from build123d import *

# Parameters (mm, degrees)
SKETCH1_W              = 55
SKETCH1_H              = 20
BOSS_EXTRUDE2_DEPTH    = 40
FILLET3_R              = 27.5
SKETCH3_R              = 10.2
CUT_EXTRUDE1_DEPTH     = 40
SKETCH4_R              = 1.5
CUT_EXTRUDE2_DEPTH     = 40
CUT_EXTRUDE3_OUTLINE_W = 1.013964341
CUT_EXTRUDE3_OUTLINE_H = 3.461369181
CUT_EXTRUDE4_OUTLINE_W = 1.011767624
CUT_EXTRUDE4_OUTLINE_H = 3.485879142


# Read off the part's stored shape, not the designer's step: Cut-Extrude3, Cut-Extrude4
with BuildPart() as part:
    # Sketch1 → Boss-Extrude2 (new body)
    with BuildSketch(Plane(origin=(0, 0, 0), x_dir=(1, 0, 0), z_dir=(0, 1, 0))):
        Rectangle(SKETCH1_W, SKETCH1_H)
    extrude(amount=BOSS_EXTRUDE2_DEPTH)

    # Fillet3
    fillet3_edges = [part.edges().sort_by_distance(p)[0] for p in [
        (27.5, 40, 0),
        (-27.5, 40, 0),
    ]]
    fillet(fillet3_edges, radius=FILLET3_R - 0.0001)  # a hair under: the kernel refuses the full size

    # Sketch3 → Cut-Extrude1 (cut)
    with BuildSketch(Plane(origin=(0, 0, -10), x_dir=(-1, 0, 0), z_dir=(0, 0, -1))):
        with Locations((0, 20)):
            Circle(SKETCH3_R)
    extrude(amount=-CUT_EXTRUDE1_DEPTH, mode=Mode.SUBTRACT)

    # Sketch4 → Cut-Extrude2 (cut)
    with BuildSketch(Plane.XZ):
        with Locations(Location((-11.5, 0, 0), (0, 0, 270))):
            Circle(SKETCH4_R)
        with Locations(Location((11.5, 0, 0), (0, 0, 270))):
            Circle(SKETCH4_R)
    extrude(amount=-CUT_EXTRUDE2_DEPTH, mode=Mode.SUBTRACT)

    # Cut-Extrude3 outline → Cut-Extrude3 (revolve, cut)
    with BuildSketch(Plane(origin=(11.536337156, 0, 0.030463059), x_dir=(1, 0, 0), z_dir=(0, 0, 1))):
        with Locations((1.959565013, 36.730684591)):
            Rectangle(CUT_EXTRUDE3_OUTLINE_W, CUT_EXTRUDE3_OUTLINE_H)
    revolve(axis=Axis((11.536337156, 0, 0.030463059), (0, 1, 0)), mode=Mode.SUBTRACT)

    # Cut-Extrude4 outline → Cut-Extrude4 (revolve, cut)
    with BuildSketch(Plane(origin=(-11.463662844, 0, 0.030463059), x_dir=(1, 0, 0), z_dir=(0, 0, 1))):
        with Locations((1.958466654, 36.742939571)):
            Rectangle(CUT_EXTRUDE4_OUTLINE_W, CUT_EXTRUDE4_OUTLINE_H)
    revolve(axis=Axis((-11.463662844, 0, 0.030463059), (0, 1, 0)), mode=Mode.SUBTRACT)


solid = part.part
Input: part model. Units: mm. Frame: model coordinates. A direction names the side the tool comes from. Give positions to 0.01 mm unless a question says otherwise; leave off trailing zeros. Loops run counter-clockwise (first coordinate to the right, second up) from the corner with the lowest first, then second, coordinate; pieces in that order, holes last. Notation, with made-up numbers: M 20.25,39.25 L 34.25,39.25 A24 cw 34.25,62.25 Z; hole C 0,-0.75 d1. An arc over 180 degrees is marked long. Use one line per item in the form item = value.
1. Section query D-D, the plane y = 32.5. Return the cut outline in (x, z).
Numbers:
outline = M -18.87,-10 L 18.87,-10 L 18.87,10 L -18.87,10 Z; hole C -11.5,0 d3; hole C 11.5,0 d3
2. Line query: L1, parallel to X at y = 9, z = 0; L2, parallel to X at y = 27.5, z = -7; L3, parallel to Y at x = -11.5, z = 1.75. Output: solid intervals per line, ascending.
Numbers:
L1 = -27.5 to -13, -10 to 10, 13 to 27.5
L2 = -23.05 to -6.91, 6.91 to 23.05
L3 = 0 to 35
3. Pull-direction query (Z, two-part tool) for faces 1 (the face through (13, 35, 1)), 2 (the face through (-27.5, 6, 0)), 3 (the face through (6, 11, 10)); classes: released by +Z, released by -Z, zero draft, split by the parting line, or undercut.
Numbers:
face_1 = undercut
face_2 = zero draft
face_3 = released by +Z
4. Reachability of faces 4 (the face through (-13, 35, -1)), 5 (the face through (-13, 17, 0)) from +Z, -Z, +X, -X, +Y, -Y: full face, straight path, thin tool, end or side. Return the list, or none.
Numbers:
face_4 = +Y
face_5 = +Y, -Y
5. Section query C-C, the plane y = 21.5. Return the cut outline in (x, z).
Numbers:
outline = M -25.99,-10 L -10.09,-10 L -10.09,-0.51 A1.5 cw long -10.09,0.51 L -10.09,10 L -25.99,10 Z; M 10.09,-10 L 25.99,-10 L 25.99,10 L 10.09,10 L 10.09,0.51 A1.5 cw long 10.09,-0.51 Z
6. Section query A-A, the plane x = -11.5. Return the cut outline in (y, z).
Numbers:
outline = M 0,-10 L 37.48,-10 L 37.48,-2.43 L 35,-2.43 L 35,-1.5 L 0,-1.5 Z; M 0,1.5 L 35,1.5 L 35,2.49 L 37.48,2.49 L 37.48,10 L 0,10 Z
7. First-contact query: pin 1 (5.5 mm diameter, centred on x = -10.5, z = 0.5, fed in from +Y); pin 2 (3.5 mm diameter, centred on x = -11.5, z = 0, fed in from +Y); pin 3 (4 mm diameter, centred on y = 24.5, z = 1.5, fed in from +X). Flat tips, straight axial feed; report the tip coordinate or a pass-through.
Numbers:
pin_1 = 38.89
pin_2 = 35
pin_3 = 25.62
